from build123d import *

# Parameters (mm, degrees)
BOSS_EXTRUDE1_DEPTH = 274


with BuildPart() as part:
    # Sketch1 → Boss-Extrude1 (new body)
    with BuildSketch(Plane.XY):
        with BuildLine():
            Line((0, 0), (0, 62))
            ThreePointArc((0, 62), (5.272077939, 74.727922061), (18, 80))
            Line((18, 80), (80, 80))
            Line((80, 80), (80, 82))
            Line((80, 82), (18, 82))
            ThreePointArc((18, 82), (3.857864376, 76.142135624), (-2, 62))
            Line((-2, 62), (-2, 0))
            Line((-2, 0), (0, 0))
        make_face()
    extrude(amount=-BOSS_EXTRUDE1_DEPTH)


solid = part.part
Here's how the part is built. I have some questions about the finished solid (model axes, mm). A direction names the side the tool comes from. Round coordinates to 2 decimals unless told otherwise and drop trailing zeros. Write each loop counter-clockwise with the first axis right and the second up, starting at its lowest first coordinate (ties: lowest second). Pieces come first, ordered by that corner, then holes. Notation, with made-up numbers: (7, -27.5) -> (38, -27.5) arc R5 ccw to (38, -22.5) -> close; hole circle Ø1 at (80.25, 42.5). An arc over 180 degrees is marked (long way). One line per item, written item: value.
1) Suppose I cut it at C-C on y = 31. List the corners of the cut face in (x, z) for me.
Filled sheet:
outline: (-2, -274) -> (0, -274) -> (0, 0) -> (-2, 0) -> close
2) Suppose I cut it at B-B on x = 68. List the corners of the cut face in (y, z) for me.
Filled sheet:
outline: (80, -274) -> (82, -274) -> (82, 0) -> (80, 0) -> close
3) For faces 1 (the face through (4.014, 76.297, -135.082)), 2 (the face through (49, 80, -135)), which set-ups out of +Z, -Z, +X, -X, +Y, -Y let a thin tool reach every point of the face, with its end or its side?
Filled sheet:
face 1: +Z, -Z, -X, +Y
face 2: +Z, -Z, +X, -Y
4) I'm going to push flat-ended pins straight in: pin 1 Ø1 at (y, z) = (72, -50.5) entering from -X; pin 2 Ø1.5 at (x, z) = (28, -80) entering from -Y. Where does each tip first touch, or does it pass through?
Filled sheet:
pin 1: stops at x = 0.4
pin 2: stops at y = 80
5) If I drill on line 1 (Y direction, x = 58, z = -240); line 2 (X direction, y = 52, z = -202); line 3 (X direction, y = 69, z = -117.5) (3 decimals), over which ranges is the centre line in solid material (lowest first)? Write a range as [from, to].
Filled sheet:
line 1: y = [80, 82]
line 2: x = [-2, 0]
line 3: x = [-0.735, 1.417]
6) Suppose I cut it at A-A on z = -30. List the corners of the cut face in (x, y) for me, plus the area to 3 significant figures.
Filled sheet:
outline: (-2, 0) -> (0, 0) -> (0, 62) arc R18 cw to (18, 80) -> (80, 80) -> (80, 82) -> (18, 82) arc R20 ccw to (-2, 62) -> close
area: 308 mm2
